Design review of the part built by this model. Coordinates are the model's own, in mm. A direction names the side the tool comes from. Round coordinates to 2 decimals unless told otherwise and drop trailing zeros. Order: outer loops, then holes, each group sorted by start corner. A loop starts at its lowest first (then second) coordinate and runs counter-clockwise, first axis right, second up.
from build123d import *

# Parameters (mm, degrees)
BOSS_EXTRUDE1_DEPTH  = 30
SHELL1_START         = 4
SHELL1_OUTLINE_W     = 23
SHELL1_OUTLINE_H     = 26
SHELL1_DEPTH         = 22
SKETCH2_W            = 9
SKETCH2_H            = 9
BOSS_EXTRUDE2_DEPTH  = 2
SKETCH3_W            = 9
SKETCH3_H            = 9
BOSS_EXTRUDE3_DEPTH  = 2
BOSS_EXTRUDE4_START  = -15.556349
SKETCH4_R            = 2.25
BOSS_EXTRUDE4_DEPTH  = 15.556349
M6_CLEARANCE_HOLE2_D = 6.6
M6_CLEARANCE_HOLE3_D = 6.6


# Read off the part's stored shape, not the designer's step: Shell1
with BuildPart() as part:
    # Sketch1 → Boss-Extrude1 (new body)
    with BuildSketch(Plane.XY):
        Polygon((0, 0), (30, 0), (0, 30), align=None)
    extrude(amount=-BOSS_EXTRUDE1_DEPTH)

    # Shell1 outline → Shell1 (cut)
    with BuildSketch(Plane.YZ.offset(SHELL1_START)):
        with Locations((15.5, -15)):
            Rectangle(SHELL1_OUTLINE_W, SHELL1_OUTLINE_H)
    extrude(amount=SHELL1_DEPTH, mode=Mode.SUBTRACT)

    # Sketch2 → Boss-Extrude2 (add)
    with BuildSketch(Plane(origin=(0, 4, 0), x_dir=(1, 0, 0), z_dir=(0, 1, 0))):
        with Locations((15, 15)):
            Rectangle(SKETCH2_W, SKETCH2_H)
    extrude(amount=BOSS_EXTRUDE2_DEPTH)

    # Sketch3 → Boss-Extrude3 (add)
    with BuildSketch(Plane(origin=(4, 0, 0), x_dir=(0, 0, -1), z_dir=(1, 0, 0))):
        with Locations((15, 15)):
            Rectangle(SKETCH3_W, SKETCH3_H)
    extrude(amount=BOSS_EXTRUDE3_DEPTH)

    # Sketch4 → Boss-Extrude4 (add)
    # profile 1 of 2: a face of its own
    with BuildSketch(Plane(origin=(15, 15, 0), x_dir=(0, 0, -1), z_dir=(0.7071067811865477, 0.7071067811865475, 0)).offset(BOSS_EXTRUDE4_START)):
        with BuildLine():
            Line((2, 3), (2, -3))
            Line((2, -3), (5, -3))
            ThreePointArc((5, -3), (8, 0), (5, 3))
            Line((5, 3), (2, 3))
        make_face()
        with Locations(Location((5, 0, 0), (0, 0, 90))):
            Circle(SKETCH4_R, mode=Mode.SUBTRACT)
    # profile 2 of 2: a face of its own
    with BuildSketch(Plane(origin=(15, 15, 0), x_dir=(0, 0, -1), z_dir=(0.7071067811865477, 0.7071067811865475, 0)).offset(BOSS_EXTRUDE4_START)):
        with BuildLine():
            Line((25, -3), (28, -3))
            Line((28, -3), (28, 3))
            Line((28, 3), (25, 3))
            ThreePointArc((25, 3), (22, 0), (25, -3))
        make_face()
        with Locations(Location((25, 0, 0), (0, 0, 90))):
            Circle(SKETCH4_R, mode=Mode.SUBTRACT)
    extrude(amount=BOSS_EXTRUDE4_DEPTH)

    # M6 Clearance Hole2 (through all)
    with Locations(Plane(origin=(0, 6, 0), x_dir=(1, 0, 0), z_dir=(0, 1, 0))):
        with Locations((15, 15)):
            Hole(M6_CLEARANCE_HOLE2_D / 2)

    # M6 Clearance Hole3 (through all)
    with Locations(Plane(origin=(6, 0, 0), x_dir=(0, 0, -1), z_dir=(1, 0, 0))):
        with Locations((15, 15)):
            Hole(M6_CLEARANCE_HOLE3_D / 2)


solid = part.part
1) Clearance check with flat-ended pins moving along their axes: P1, Ø6, axis at x = 5, z = -10.5, coming from the +Y side; P2, Ø1.6, axis at x = 5, z = -14.5, coming from the +Y side; P3, Ø11, axis at y = 13, z = -9.5, coming from the +X side; P4, Ø5.5, axis at y = 15, z = -15, coming from the -X side. State where each tip first meets the part, or that it passes through.
Results:
P1: stops at y = 28
P2: stops at y = 19.5
P3: stops at x = 17.12
P4: passes through
2) Take a section at C-C on z = -20.25. Give the boundary of the cut face in (x, y), plus the area to 3 significant figures.
Results:
outline: (0, 0) - (30, 0) - (26, 4) - (4, 4) - (4, 26) - (0, 30) - close
area: 208 mm2
3) Take a section at D-D on x = 27. Give the boundary of the cut face in (y, z), plus the area to 3 significant figures.
Results:
outline: (0, -30) - (3, -30) - (3, 0) - (0, 0) - close
area: 90.0 mm2
4) Take a section at B-B on x = 3.5. Give the boundary of the cut face in (y, z).
Results:
outline: (0, -30) - (26.5, -30) - (26.5, 0) - (0, 0) - close; hole circle Ø6.6 at (15, -15)
5) For faces 1 (the face through (5, 15, -19.5)), 2 (the face through (20, 4, -15)), 3 (the face through (17, 7, -28)), list the 3-axis set-ups (+Z, -Z, +X, -X, +Y, -Y) from which the entire face can be reached by the end or side of a thin tool; tool diameter is ignored.
Results:
face 1: +X, +Y
face 2: none
face 3: +X
6) Take a section at A-A on z = -15. Give the boundary of the cut face in (x, y), plus the area to 3 significant figures.
Results:
outline: (0, 0) - (11.7, 0) - (11.7, 6) - (10.5, 6) - (10.5, 4) - (4, 4) - (4, 10.5) - (6, 10.5) - (6, 11.7) - (0, 11.7) - close; (0, 18.3) - (6, 18.3) - (6, 19.5) - (4, 19.5) - (4, 26) - (0, 30) - close; (18.3, 0) - (30, 0) - (26, 4) - (19.5, 4) - (19.5, 6) - (18.3, 6) - close
area: 165 mm2
7) The part is to be moulded in two halves that separate along Z. For faces 4 (the face through (4, 5, -5)), 5 (the face through (15, 15, -28)), 6 (the face through (8, 9, -30)), say which applies: released by +Z, released by -Z, zero draft, split by the parting line, or undercut.
Results:
face 4: undercut
face 5: zero draft
face 6: released by -Z
8) To check wall thickness, follow line 1 along Z through (x, y) = (11, 5.5); line 2 along X through (y, z) = (11.5, -26.25); line 3 along Z through (x, y) = (8.5, 6). State the ranges of each line that lie inside material, in increasing order.
Results:
line 1: z = -30 to -28, -19.5 to -10.5, -2 to 0
line 2: x = 0 to 4, 7.26 to 8.85, 14.15 to 15.74
line 3: z = -30 to -26.39, -23.61 to -22.58, -7.42 to -6.39, -3.61 to 0
